```python
from build123d import *

# Parameters (mm, degrees)
AUFSATZ_LINEAR_AUSTRAGEN1_DEPTH = 50
SKIZZE2_R                       = 16
SCHNITT_LINEAR_AUSTRAGEN1_DEPTH = 50


with BuildPart() as part:
    # Skizze1 → Aufsatz-Linear austragen1 (new body)
    with BuildSketch(Plane.XY):
        Polygon((0, 65), (8, 65), (8, 10), (65, 10), (65, 0), (0, 0), align=None)
    extrude(amount=-AUFSATZ_LINEAR_AUSTRAGEN1_DEPTH)

    # Skizze2 → Schnitt-Linear austragen1 (cut)
    with BuildSketch(Plane(origin=(8, 0, 0), x_dir=(0, 0, -1), z_dir=(1, 0, 0))):
        with Locations((25, 37.5)):
            Circle(SKIZZE2_R)
    extrude(amount=-SCHNITT_LINEAR_AUSTRAGEN1_DEPTH, mode=Mode.SUBTRACT)


solid = part.part
```
Geometry: final body of the model. Coordinates: model frame, mm. A direction names the side the tool comes from. Round coordinates to 2 decimals unless told otherwise and drop trailing zeros. Order: outer loops, then holes, each group sorted by start corner. A loop starts at its lowest first (then second) coordinate and runs counter-clockwise, first axis right, second up. Notation, with made-up numbers: M 26,63 L 66,63 A22 ccw 66,86 Z; hole C 56.25,39.5 d6. An arc over 180 degrees is marked long. One line per item, written item: value.
(1) Cut plane B-B (z = -35). Return the cut outline in (x, y).
Result sheet:
outline: M 0,0 L 65,0 L 65,10 L 8,10 L 8,25.01 L 0,25.01 Z; M 0,49.99 L 8,49.99 L 8,65 L 0,65 Z
(2) Cut plane C-C (z = -44). Return the cut outline in (x, y).
Result sheet:
outline: M 0,0 L 65,0 L 65,10 L 8,10 L 8,65 L 0,65 Z
(3) Pin query (flat end, axial travel): P1, Ø3, axis at x = 35.5, z = -15, coming from the +Y side; P2, Ø10, axis at y = 30, z = -37, coming from the +X side. Return the tip coordinate at first contact, or that it passes through.
Result sheet:
P1: y = 10
P2: x = 8
(4) Reachability of faces 4 (the flat face through (36, 10, -25)), 5 (the flat face through (21, 9, 0)) from +Z, -Z, +X, -X, +Y, -Y: full face, straight path, thin tool, end or side. Return the list, or none.
Result sheet:
face 4: +Z, -Z, +X, +Y
face 5: +Z, +X, -X, +Y, -Y
(5) Cut plane D-D (y = 47). Return the cut outline in (x, z).
Result sheet:
outline: M 0,-50 L 8,-50 L 8,-37.87 L 0,-37.87 Z; M 0,-12.13 L 8,-12.13 L 8,0 L 0,0 Z
(6) Line query: probe 1 along Y at (x, z) = (6, -25); probe 2 along Z at (x, y) = (6, 37); probe 3 along Y at (x, z) = (37.5, -17). Output: solid intervals per line, ascending. Write a range as [from, to].
Result sheet:
probe 1: [0, 21.5], [53.5, 65]
probe 2: [-50, -40.99], [-9.01, 0]
probe 3: [0, 10]
(7) Cut plane A-A (y = 37.5). Return the cut outline in (x, z), and give its area (3 significant figures).
Result sheet:
outline: M 0,-50 L 8,-50 L 8,-41 L 0,-41 Z; M 0,-9 L 8,-9 L 8,0 L 0,0 Z
area: 144 mm2
(8) Pull-direction query (Y, two-part tool) for faces 1 (the flat face through (0, 25, -14)), 2 (the cylindrical face through (4.06, 42.31, -40.26)), 3 (the flat face through (33, 0, -25)); classes: pulls with the +Y half, pulls with the -Y half, needs draft (parallel to the pull), parting line crosses it, or undercut.
Result sheet:
face 1: needs draft
face 2: undercut
face 3: pulls with the -Y half
